from build123d import *

# Parameters (mm, degrees)
SKETCH1_R               = 19
BOSS_EXTRUDE1_DEPTH     = 34.5
SKETCH2_R               = 10
BOSS_EXTRUDE2_DEPTH     = 5
SKETCH3_R               = 3
BOSS_EXTRUDE3_DEPTH     = 15
SKETCH4_W               = 10
SKETCH4_H               = 0.65
CUT_EXTRUDE1_DEPTH      = 20
CUT_EXTRUDE1_DEPTH_BACK = 20
FILLET1_R               = 2
SKETCH5_R               = 1.5
CUT_EXTRUDE2_DEPTH      = 3


with BuildPart() as part:
    # Sketch1 → Boss-Extrude1 (new body)
    with BuildSketch(Plane.XY):
        Circle(SKETCH1_R)
    extrude(amount=BOSS_EXTRUDE1_DEPTH)

    # Sketch2 → Boss-Extrude2 (add)
    with BuildSketch(Plane.XY.offset(34.5)):
        Circle(SKETCH2_R)
    extrude(amount=BOSS_EXTRUDE2_DEPTH)

    # Sketch3 → Boss-Extrude3 (add)
    with BuildSketch(Plane.XY.offset(39.5)):
        Circle(SKETCH3_R)
    extrude(amount=BOSS_EXTRUDE3_DEPTH)

    # Sketch4 → Cut-Extrude1 (cut, two sides)
    with BuildSketch(Plane(origin=(0, 0, 0), x_dir=(0, 0, -1), z_dir=(1, 0, 0))) as cut_extrude1_sk:
        with Locations((-49.5, 2.675)):
            Rectangle(SKETCH4_W, SKETCH4_H)
    extrude(amount=CUT_EXTRUDE1_DEPTH, mode=Mode.SUBTRACT)
    extrude(cut_extrude1_sk.sketch, amount=-CUT_EXTRUDE1_DEPTH_BACK, mode=Mode.SUBTRACT)

    # Fillet1
    fillet1_edges = [part.edges().sort_by_distance(p)[0] for p in [
        (-19, 0, 0),
    ]]
    fillet(fillet1_edges, radius=FILLET1_R)

    # Sketch5 → Cut-Extrude2 (cut)
    with BuildSketch(Plane.XY.offset(34.5)):
        with Locations((0, 15)):
            Circle(SKETCH5_R)
        with Locations((12.990381057, -7.5)):
            Circle(SKETCH5_R)
        with Locations((-12.990381057, -7.5)):
            Circle(SKETCH5_R)
    extrude(amount=-CUT_EXTRUDE2_DEPTH, mode=Mode.SUBTRACT)


solid = part.part
The listing builds one solid part. Answer for the finished solid, in the listing's coordinates (mm). A direction names the side the tool comes from. Give positions to 0.01 mm unless a question says otherwise; leave off trailing zeros. Order: outer loops, then holes, each group sorted by start corner. A loop starts at its lowest first (then second) coordinate and runs counter-clockwise, first axis right, second up. Notation, with made-up numbers: (37.25, 37) - (87.25, 37) arc R17 ccw to (87.25, 56) - close; hole circle Ø5 at (-3, 14). An arc over 180 degrees is marked (long way). One line per item, written item: value. Start each with the question number.
1) The mould has two halves that part along X. Classify faces 3 (the face through (13, -7, 31.5)), 4 (the face through (-1.11, 16.01, 33.02)), 5 (the face through (0, 2.35, 50)), 6 (the face through (-2.17, -9.76, 36.97)): released by +X, released by -X, zero draft, split by the parting line, or undercut.
2) Given pin 1 Ø4 at (x, y) = (-6, 0) entering from +Z; pin 2 Ø4 at (x, y) = (12.99, -7.5) entering from -Z; pin 3 Ø4 at (y, z) = (2, 38) entering from -X; pin 4 Ø4 at (x, z) = (11.5, 29) entering from +Y, each flat-ended and moving along its own axis, determine where each tip first touches the part or whether it passes through.
3) A cutting plane is placed at A-A on y = 0. Give the vertices of the cut face in (x, z), then the cut area to 3 significant figures.
4) A tool of negligible diameter and unlimited length cuts with its end or side. For faces 1 (the face through (-13, -7, 31.5)), 2 (the face through (8.767, -16.856, 18.022)), from which of +Z, -Z, +X, -X, +Y, -Y can it reach the whole face along a straight path? Write none if from no direction.
5) A cutting plane is placed at D-D on z = 33.5. Give the vertices of the cut face in (x, y).
6) Find the intervals of material crossed by L1, parallel to Y at x = 0, z = 32.4; L2, parallel to X at y = -7, z = 32; L3, parallel to Z at x = 3, y = 3, in increasing order.
7) A cutting plane is placed at B-B on x = 0. Give the vertices of the cut face in (y, z), then the cut area to 3 significant figures.
8) A cutting plane is placed at C-C on z = 4.5. Give the vertices of the cut face in (x, y).
Answer sheet:
1. face 3: undercut
1. face 4: undercut
1. face 5: zero draft
1. face 6: split by the parting line
2. pin 1: stops at z = 39.5
2. pin 2: stops at z = 0
2. pin 3: stops at x = -10
2. pin 4: stops at y = 16.45
3. outline: (-19, 2) arc R2 ccw to (-17, 0) - (17, 0) arc R2 ccw to (19, 2) - (19, 34.5) - (10, 34.5) - (10, 39.5) - (3, 39.5) - (3, 54.5) - (-3, 54.5) - (-3, 39.5) - (-10, 39.5) - (-10, 34.5) - (-19, 34.5) - close
3. area: 1,500 mm2
4. face 1: +Z
4. face 2: +Z, -Z
5. outline: circle Ø38 at (0, 0); hole circle Ø3 at (-12.99, -7.5); hole circle Ø3 at (0, 15); hole circle Ø3 at (12.99, -7.5)
6. L1: y = -19 to 13.5, 16.5 to 19
6. L2: x = -17.66 to -14.4, -11.58 to 11.58, 14.4 to 17.66
6. L3: z = 0 to 39.5
7. outline: (-19, 2) arc R2 ccw to (-17, 0) - (17, 0) arc R2 ccw to (19, 2) - (19, 34.5) - (16.5, 34.5) - (16.5, 31.5) - (13.5, 31.5) - (13.5, 34.5) - (10, 34.5) - (10, 39.5) - (3, 39.5) - (3, 44.5) - (2.35, 44.5) - (2.35, 54.5) - (-3, 54.5) - (-3, 39.5) - (-10, 39.5) - (-10, 34.5) - (-19, 34.5) - close
7. area: 1,480 mm2
8. outline: circle Ø38 at (0, 0)
